Geometry check sheet. Reference: the model listing, model coordinates, mm. A direction names the side the tool comes from. Give positions to 0.01 mm unless a question says otherwise; leave off trailing zeros. Write each loop counter-clockwise with the first axis right and the second up, starting at its lowest first coordinate (ties: lowest second). Pieces come first, ordered by that corner, then holes. Notation, with made-up numbers: M 15.5,61 L 72.5,61 A5 cw 72.5,66 Z; hole C -1.5,76.5 d10. An arc over 180 degrees is marked long. Write each question's results on one line, items separated by ' | '.
```python
from build123d import *

# Parameters (mm, degrees)
F0_W     = 19
F0_H     = 19
F1_DEPTH = 19
F2_R     = 8.5
F5_DEPTH = 25
F3_R     = 8.5
F6_DEPTH = 25
F4_R     = 8.5
F7_DEPTH = 25
F8_R     = 2
F9_R     = 7
F10_SIZE = 0.99999
F11_SIZE = 0.99999
F12_SIZE = 0.99999


# Not quite as in the source:
# - a fillet or chamfer is up to 0.001 mm smaller than in the source, because OpenCascade refuses the exact size


with BuildPart() as f1:
    # F0 (on Top) → F1 (new body)
    with BuildSketch(Plane.XY):
        with Locations((-4.8786746205, -4.1296786368)):
            Rectangle(F0_W, F0_H)
    extrude(amount=F1_DEPTH)

    # F2 (on face) → F5 (join)
    with BuildSketch(Plane.XZ.offset(13.6296786368)):
        with Locations((-4.8786746205, 9.5)):
            Circle(F2_R)
    extrude(amount=F5_DEPTH)

    # F3 (on face) → F6 (join)
    with BuildSketch(Plane.YZ.offset(4.6213253795)):
        with Locations((-4.1296786368, 9.5)):
            Circle(F3_R)
    extrude(amount=F6_DEPTH)

    # F4 (on face) → F7 (join)
    with BuildSketch(Plane.XY.offset(19)):
        with Locations((-4.8786746205, -4.1296786368)):
            Circle(F4_R)
    extrude(amount=F7_DEPTH)

    # F8
    f8_edges = [f1.edges().sort_by_distance(p)[0] for p in [
        (-13.378675, -38.629679, 9.5),
        (29.621325, -12.629679, 9.5),
        (-13.378675, -4.129679, 44),
    ]]
    fillet(f8_edges, radius=F8_R)

    # F9
    f9_edges = [f1.edges().sort_by_distance(p)[0] for p in [
        (-14.378675, 5.370321, 9.5),
    ]]
    fillet(f9_edges, radius=F9_R)

    # F10 (size 1 in the source; OpenCascade refuses exactly that, so slightly less here)
    f10_edges = [f1.edges().sort_by_distance(p)[0] for p in [
        (4.621325, -4.129679, 19),
    ]]
    chamfer(f10_edges, length=F10_SIZE)

    # F11 (size 1 in the source; OpenCascade refuses exactly that, so slightly less here)
    f11_edges = [f1.edges().sort_by_distance(p)[0] for p in [
        (4.621325, -13.629679, 9.000005),
        (4.12133, -13.629679, 18.500005),
        (-5.37867, -13.629679, 19),
    ]]
    chamfer(f11_edges, length=F11_SIZE)

    # F12 (call 1 of 2: OpenCascade refuses the feature's edges together) (size 1 in the source; OpenCascade refuses exactly that, so slightly less here)
    f12_edges = [f1.edges().sort_by_distance(p)[0] for p in [
        (-1.87867, 5.370321, 19),
        (-12.328422, 3.320069, 19),
        (-14.378675, -7.129684, 19),
        (-14.378675, -13.629679, 9.000005),
        (-14.378675, -13.129684, 18.500005),
    ]]
    chamfer(f12_edges, length=F12_SIZE)

    # F12#2 (call 2 of 2) (size 1 in the source; OpenCascade refuses exactly that, so slightly less here)
    f12_2_edges = [f1.edges().sort_by_distance(p)[0] for p in [
        (4.621325, 5.370321, 9.000005),
    ]]
    chamfer(f12_2_edges, length=F12_SIZE)


solid = f1.part
```
Q1. Material ranges on probe 1 along Y at (x, z) = (26, 10); probe 2 along Z at (x, y) = (2, 3.5); probe 3 along X at (y, z) = (-11, 18), recorded low to high. Write a range as [from, to].
Answer key:
probe 1: y = [-12.61, 4.36] | probe 2: z = [0, 19] | probe 3: x = [-14.38, 4.62]
Q2. Section check C-C (y = -21). Enter the section's corners in (x, z), then the cut area to 3 significant figures.
Answer key:
outline: C -4.88,9.5 d17 | area: 227 mm2
Q3. Section check B-B (x = 7.5). Enter the section's corners in (y, z).
Answer key:
outline: C -4.13,9.5 d17
Q4. Depth check by flat-ended pin: P1, Ø4, axis at y = -20.5, z = 6, coming from the +X side; P2, Ø2, axis at x = -7, y = -27, coming from the -Z side; P3, Ø1, axis at y = -16.5, z = 7.5, coming from the -X side; P4, Ø12, axis at y = -12, z = 19.5, coming from the -X side. Enter the tip coordinate at first touch or a pass-through.
Answer key:
P1: stops at x = 3.49 | P2: stops at z = 1.07 | P3: stops at x = -13.25 | P4: stops at x = -14.38
Q5. Access from +Z, -Z, +X, -X, +Y, -Y to the whole of each face (thin tool, end or side, straight path). Record for faces 1 (the face through (15.96, -5.97, 1.2)), 2 (the face through (-11.624, -9.302, 30.339)), 3 (the face through (-12.38, 3.27, 9.13)), 4 (the face through (-2, 5.37, 9)), 5 (the face through (-7, -13.63, 1)).
Answer key:
face 1: +X | face 2: +Z | face 3: +Z, -Z, -X, +Y | face 4: +Z, -Z, +X, -X, +Y | face 5: -Y
